from build123d import *

# Parameters (mm, degrees)
SKETCH1_W           = 100.85
SKETCH1_H           = 70.53
BOSS_EXTRUDE1_DEPTH = 2
SKETCH6_W           = 104.85
SKETCH6_H           = 74.53
BOSS_EXTRUDE3_DEPTH = 2
SKETCH3_R           = 2.5
BOSS_EXTRUDE2_DEPTH = 5
FILLET1_SIZE        = 1.5
FILLET1_SIZE_2      = 4
FILLET2_R           = 4


with BuildPart() as part:
    # Sketch1 → Boss-Extrude1 (new body)
    with BuildSketch(Plane.XY):
        with Locations((0.782139599, -9.454393248)):
            Rectangle(SKETCH1_W, SKETCH1_H)
    extrude(amount=BOSS_EXTRUDE1_DEPTH)

    # Sketch6 → Boss-Extrude3 (add)
    with BuildSketch(Plane.XY.offset(2)):
        with Locations((0.782139599, -9.454393248)):
            Rectangle(SKETCH6_W, SKETCH6_H)
    extrude(amount=-BOSS_EXTRUDE3_DEPTH)

    # Sketch3 → Boss-Extrude2 (add)
    with BuildSketch(Plane.XY.offset(2)):
        with Locations((-29.192860401, 22.360606752)):
            Circle(SKETCH3_R)
    boss_extrude2 = extrude(amount=BOSS_EXTRUDE2_DEPTH)

    # Sketch5 → Tap Drill for M3x0.5 Tap1 (revolve, cut)
    with BuildSketch(Plane(origin=(-29.192860401, 22.360606752, 7), x_dir=(0, -1, 0), z_dir=(1, 0, 0))):
        Polygon((0, 0), (0, 10.751075774), (1.25, 10), (1.25, 0), align=None)
    tap_drill_for_m3x0_5_tap1 = revolve(axis=Axis((-29.192860401, 22.360606752, 13.35), (0, 0, -1)), mode=Mode.SUBTRACT)

    # Sketch-Pattern1: Boss-Extrude2, Tap Drill for M3x0.5 Tap1 at 4 more places
    with Locations((-17.86, -34.92, 0), (13.94, -37.51, 0), (77.82, -64.41, 0), (62.15, 0.23, 0)):
        add(boss_extrude2)
        add(tap_drill_for_m3x0_5_tap1, mode=Mode.SUBTRACT)

    # Fillet1
    # an asymmetric fillet: 4, 1.5 mm, written as the material it adds along each edge
    with BuildSketch(Plane(origin=(-29.192860401, 22.360606752, 2), x_dir=(1, 0, 0), z_dir=(0, -1, 0))) as fillet1_piece_1:
        with BuildLine():
            Bezier((2.5 + FILLET1_SIZE, 0), (2.5, 0), (2.5, FILLET1_SIZE_2), weights=[1, 0.707106781, 1])
            Line((2.5, FILLET1_SIZE_2), (2.5, 0))
            Line((2.5, 0), (2.5 + FILLET1_SIZE, 0))
        make_face()
    revolve(axis=Axis((-29.192860401, 22.360606752, 2), (0, 0, 1)))
    with BuildSketch(Plane(origin=(-47.052860401, -12.559393248, 2), x_dir=(1, 0, 0), z_dir=(0, -1, 0))) as fillet1_piece_2:
        with BuildLine():
            Bezier((2.5 + FILLET1_SIZE, 0), (2.5, 0), (2.5, FILLET1_SIZE_2), weights=[1, 0.707106781, 1])
            Line((2.5, FILLET1_SIZE_2), (2.5, 0))
            Line((2.5, 0), (2.5 + FILLET1_SIZE, 0))
        make_face()
    revolve(axis=Axis((-47.052860401, -12.559393248, 2), (0, 0, 1)))
    with BuildSketch(Plane(origin=(-15.252860401, -15.149393248, 2), x_dir=(1, 0, 0), z_dir=(0, -1, 0))) as fillet1_piece_3:
        with BuildLine():
            Bezier((2.5 + FILLET1_SIZE, 0), (2.5, 0), (2.5, FILLET1_SIZE_2), weights=[1, 0.707106781, 1])
            Line((2.5, FILLET1_SIZE_2), (2.5, 0))
            Line((2.5, 0), (2.5 + FILLET1_SIZE, 0))
        make_face()
    revolve(axis=Axis((-15.252860401, -15.149393248, 2), (0, 0, 1)))
    with BuildSketch(Plane(origin=(48.627139599, -42.049393248, 2), x_dir=(1, 0, 0), z_dir=(0, -1, 0))) as fillet1_piece_4:
        with BuildLine():
            Bezier((2.5 + FILLET1_SIZE, 0), (2.5, 0), (2.5, FILLET1_SIZE_2), weights=[1, 0.707106781, 1])
            Line((2.5, FILLET1_SIZE_2), (2.5, 0))
            Line((2.5, 0), (2.5 + FILLET1_SIZE, 0))
        make_face()
    revolve(axis=Axis((48.627139599, -42.049393248, 2), (0, 0, 1)))
    with BuildSketch(Plane(origin=(32.957139599, 22.590606752, 2), x_dir=(1, 0, 0), z_dir=(0, -1, 0))) as fillet1_piece_5:
        with BuildLine():
            Bezier((2.5 + FILLET1_SIZE, 0), (2.5, 0), (2.5, FILLET1_SIZE_2), weights=[1, 0.707106781, 1])
            Line((2.5, FILLET1_SIZE_2), (2.5, 0))
            Line((2.5, 0), (2.5 + FILLET1_SIZE, 0))
        make_face()
    revolve(axis=Axis((32.957139599, 22.590606752, 2), (0, 0, 1)))

    # Fillet2
    fillet2_edges = [part.edges().sort_by_distance(p)[0] for p in [
        (-51.642860401, 27.810606752, 1),
        (53.207139599, 27.810606752, 1),
        (53.207139599, -46.719393248, 1),
        (-51.642860401, -46.719393248, 1),
    ]]
    fillet(fillet2_edges, radius=FILLET2_R)


solid = part.part
Geometry check sheet. Reference: the model listing, model coordinates, mm. A direction names the side the tool comes from. Give positions to 0.01 mm unless a question says otherwise; leave off trailing zeros. Order: outer loops, then holes, each group sorted by start corner. A loop starts at its lowest first (then second) coordinate and runs counter-clockwise, first axis right, second up.
1. Scan lines: line 1 (Z direction, x = 23, y = 19); line 2 (X direction, y = -41, z = 0.5); line 3 (Y direction, x = -27.5, z = 6). Record each from-to range of solid material in increasing order.
Completed:
line 1: z = 0 to 2
line 2: x = -51.64 to 47.95, 49.31 to 53.21
line 3: y = 20.52 to 24.2
2. Depth check by flat-ended pin: pin 1 (1.5 mm diameter, centred on x = -15.25, y = -15.15, fed in from -Z); pin 2 (2 mm diameter, centred on x = 6.5, y = -26.5, fed in from +Z); pin 3 (3 mm diameter, centred on x = -30.5, z = 4, fed in from +Y). Enter the tip coordinate at first touch or a pass-through.
Completed:
pin 1: passes through
pin 2: stops at z = 2
pin 3: stops at y = 25.48
3. Access from +Z, -Z, +X, -X, +Y, -Y to the whole of each face (thin tool, end or side, straight path). Record for faces 4 (the face through (-26.808, 23.112, 6.493)), 5 (the face through (52.004, -45.579, 0.986)).
Completed:
face 4: +Z
face 5: +Z, -Z, +X, -Y
4. Sectioned sample at A-A (y = 3.5). Record the boundary of the cut face in (x, z).
Completed:
outline: (-51.64, 0) - (53.21, 0) - (53.21, 2) - (-51.64, 2) - close
5. Sectioned sample at B-B (x = -36.5). Record the boundary of the cut face in (y, z), then the cut area to 3 significant figures.
Completed:
outline: (-46.72, 0) - (27.81, 0) - (27.81, 2) - (-46.72, 2) - close
area: 149 mm2
6. Draft check along Y on faces 1 (the face through (-50.5, -45.52, 0.99)), 2 (the face through (33.436, 21.436, 3.549)), 3 (the face through (-49.55, -12.45, 6.49)). Enter one of: pulls with the +Y half, pulls with the -Y half, needs draft (parallel to the pull), parting line crosses it, or undercut.
Completed:
face 1: pulls with the -Y half
face 2: undercut
face 3: parting line crosses it
